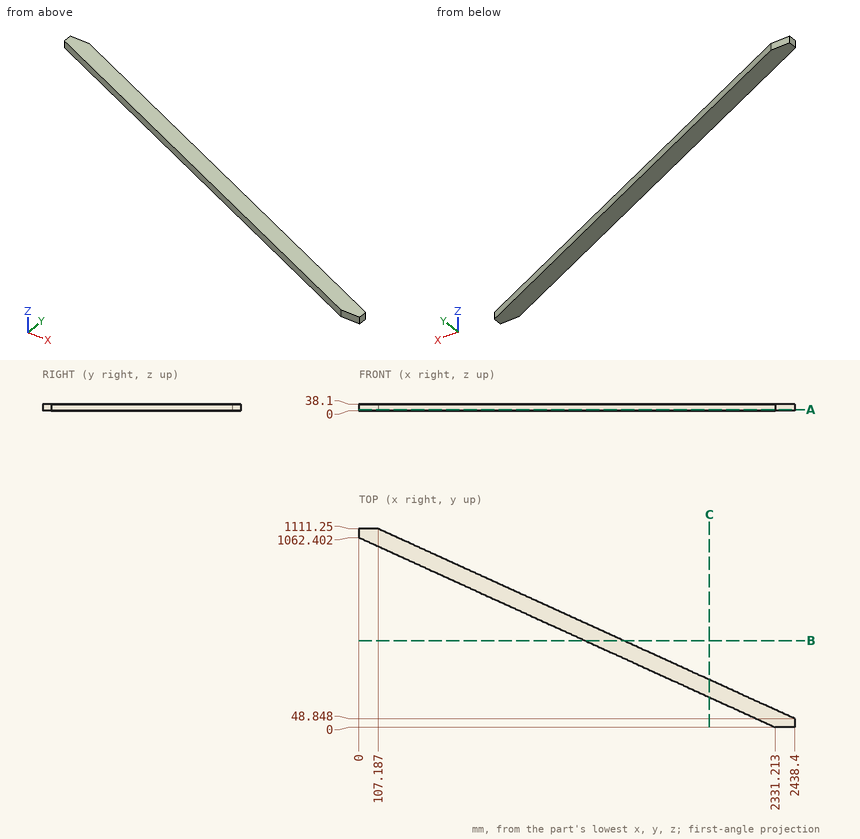
Can you work these out from the drawing? Everything is in mm from the part's minimum corner. Coordinates: 2 decimals unless noted, no trailing zeros. Loops run counter-clockwise (first coordinate to the right, second up) from the corner with the lowest first, then second, coordinate; pieces in that order, holes last. Notation, with made-up numbers: M 5.5,14 L 58.5,14 A24 cw 58.5,26 Z; hole C 43,65 d9. An arc over 180 degrees is marked long. One line per item, written item: value.
1. Please list where these lines run through material, in increasing order: probe 1 along Y at (x, z) = (1048.5, 18); probe 2 along X at (y, z) = (82.5, 29) (1 decimal); probe 3 along X at (y, z) = (997, 15) (1 decimal).
Geometry says:
probe 1: y = 584.57 to 682.27
probe 2: x = 2150.2 to 2364.6
probe 3: x = 143.5 to 357.9
2. Will these pins go through, and if not, where does the flat tip stop? pin 1 Ø6 at (y, z) = (216, 11) entering from +X (1 decimal); pin 2 Ø5 at (y, z) = (590, 16.5) entering from -X; pin 3 Ø2 at (y, z) = (190, 27.5) entering from -X (1 decimal).
Geometry says:
pin 1: stops at x = 2078.2
pin 2: stops at x = 1031.1
pin 3: stops at x = 1912.1
3. Imagine slicing it at A-A (z = 6.5). List the corners of the cut face in (x, y) for me.
Geometry says:
outline: M 0,1062.4 L 2331.21,0 L 2438.4,0 L 2438.4,48.85 L 107.19,1111.25 L 0,1111.25 Z
4. Imagine slicing it at C-C (x = 1962). List the corners of the cut face in (y, z) for me.
Geometry says:
outline: M 168.26,0 L 265.96,0 L 265.96,38.1 L 168.26,38.1 Z
5. Imagine slicing it at B-B (y = 484.5). List the corners of the cut face in (x, z) for me, and give its area (3 significant figures).
Geometry says:
outline: M 1268.08,0 L 1482.46,0 L 1482.46,38.1 L 1268.08,38.1 Z
area: 8,170 mm2
